from build123d import *

# Parameters (mm, degrees)
F0_W     = 210
F0_H     = 297
F0_W_2   = 28
F0_H_2   = 43
F1_DEPTH = 6


with BuildPart() as f1:
    # F0 (on Front) → F1 (new body)
    with BuildSketch(Plane.XZ):
        Rectangle(F0_W, F0_H)
        with Locations((-39.67, -113.3)):
            Rectangle(F0_W_2, F0_H_2, mode=Mode.SUBTRACT)
        with Locations((-39.67, -56.64)):
            Rectangle(F0_W_2, F0_H_2, mode=Mode.SUBTRACT)
        with Locations((39.66, -113.3)):
            Rectangle(F0_W_2, F0_H_2, mode=Mode.SUBTRACT)
        with Locations((39.66, -56.64)):
            Rectangle(F0_W_2, F0_H_2, mode=Mode.SUBTRACT)
        with Locations((-39.67, 0.02)):
            Rectangle(F0_W_2, F0_H_2, mode=Mode.SUBTRACT)
        with Locations((-39.67, 56.68)):
            Rectangle(F0_W_2, F0_H_2, mode=Mode.SUBTRACT)
        with Locations((-39.67, 113.34)):
            Rectangle(F0_W_2, F0_H_2, mode=Mode.SUBTRACT)
        with Locations((39.66, 0.02)):
            Rectangle(F0_W_2, F0_H_2, mode=Mode.SUBTRACT)
        with Locations((39.66, 56.68)):
            Rectangle(F0_W_2, F0_H_2, mode=Mode.SUBTRACT)
        with Locations((39.66, 113.34)):
            Rectangle(F0_W_2, F0_H_2, mode=Mode.SUBTRACT)
    extrude(amount=F1_DEPTH)


solid = f1.part
Model file for the job. Use its own axes, mm. A direction names the side the tool comes from. Give positions to 0.01 mm unless a question says otherwise; leave off trailing zeros. Loops run counter-clockwise (first coordinate to the right, second up) from the corner with the lowest first, then second, coordinate; pieces in that order, holes last.
Item 1: Slice it at C-C (y = -2.35). Give the number of separate pieces and of enclosed holes in the cut face, plus the area to 3 significant figures.
Check values:
separate pieces: 1
enclosed holes: 10
area: 50,300 mm2
Item 2: Slice it at A-A (z = 73). Write the cut outline in (x, y).
Check values:
outline: (-105, -6) - (-53.67, -6) - (-53.67, 0) - (-105, 0) - close; (-25.67, -6) - (25.66, -6) - (25.66, 0) - (-25.67, 0) - close; (53.66, -6) - (105, -6) - (105, 0) - (53.66, 0) - close
Item 3: Slice it at B-B (x = -47). Write the cut outline in (y, z).
Check values:
outline: (-6, -148.5) - (0, -148.5) - (0, -134.8) - (-6, -134.8) - close; (-6, -91.8) - (0, -91.8) - (0, -78.14) - (-6, -78.14) - close; (-6, -35.14) - (0, -35.14) - (0, -21.48) - (-6, -21.48) - close; (-6, 21.52) - (0, 21.52) - (0, 35.18) - (-6, 35.18) - close; (-6, 78.18) - (0, 78.18) - (0, 91.84) - (-6, 91.84) - close; (-6, 134.84) - (0, 134.84) - (0, 148.5) - (-6, 148.5) - close
Item 4: Which spindle directions (+Z, -Z, +X, -X, +Y, -Y) get a long thin tool onto all of the face, cutting with end or side? Do faces 1 (the face through (39, -3, 21.52)), 2 (the face through (-1, -3, -148.5)). Say none if no direction does.
Check values:
face 1: +Y, -Y
face 2: -Z, +X, -X, +Y, -Y
Item 5: Drill centre lines: line 1 along Z through (x, y) = (-36.5, -4.85); line 2 along X through (y, z) = (-2.3, -114). Where is each one in solid material? Low to high.
Check values:
line 1: z = -148.5 to -134.8, -91.8 to -78.14, -35.14 to -21.48, 21.52 to 35.18, 78.18 to 91.84, 134.84 to 148.5
line 2: x = -105 to -53.67, -25.67 to 25.66, 53.66 to 105
Item 6: Mould opens along X. For faces 3 (the face through (105, -3, -2)), 4 (the face through (-25.67, -3, 113)), 5 (the face through (-1, -6, 2)) say: +X half, -X half, draft (parallel to the pull), parting line (faces both ways), or undercut.
Check values:
face 3: +X half
face 4: undercut
face 5: draft
